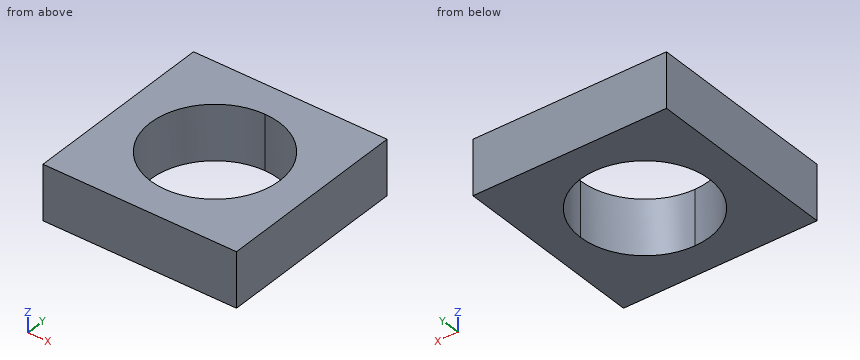
```python
from build123d import *

# Parameters (mm, degrees)
F1_DEPTH = 2.159


with BuildPart() as f1:
    # F0 (on Top) → F1 (new body)
    with BuildSketch(Plane.XY):
        with BuildLine():
            Line((-3.81, 0), (0, 0))
            Line((0, 0), (0, 1.27))
            ThreePointArc((0, 1.27), (-2.54, 3.81), (0, 6.35))
            Line((0, 6.35), (0, 7.62))
            Line((0, 7.62), (-3.81, 7.62))
            Line((-3.81, 7.62), (-3.81, 0))
        make_face()
        with BuildLine():
            Line((0, 1.27), (0, 0))
            Line((0, 0), (3.81, 0))
            Line((3.81, 0), (3.81, 7.62))
            Line((3.81, 7.62), (0, 7.62))
            Line((0, 7.62), (0, 6.35))
            ThreePointArc((0, 6.35), (1.796051, 5.606051), (2.54, 3.81))
            ThreePointArc((2.54, 3.81), (1.796051, 2.013949), (0, 1.27))
        make_face()
    extrude(amount=F1_DEPTH)


solid = f1.part
```
Could you check a few things on this model? Use its own coordinates, in mm. Round coordinates to 2 decimals unless told otherwise and drop trailing zeros. Loops run counter-clockwise (first coordinate to the right, second up) from the corner with the lowest first, then second, coordinate; pieces in that order, holes last.
Q1. I want a section at C-C (z = 1.5). Write out the boundary of the cut face in (x, y), and give its area (3 significant figures).
Q2. I want a section at B-B (x = 1). Write out the boundary of the cut face in (y, z).
Q3. Please list where these lines run through material, in increasing order: L1, parallel to Y at x = 0.5, z = 0.1; L2, parallel to X at y = 4.75, z = 0.55; L3, parallel to X at y = 3.75, z = 0.4.
Q4. I want a section at A-A (y = 3.5). Write out the boundary of the cut face in (x, z), and give its area (3 significant figures).
Answer below:
1. outline: (-3.81, 0) - (3.81, 0) - (3.81, 7.62) - (-3.81, 7.62) - close; hole (0, 6.35) arc R2.54 ccw (long way) to (2.54, 3.81) arc R2.54 ccw to start
1. area: 37.8 mm2
2. outline: (0, 0) - (1.48, 0) - (1.48, 2.16) - (0, 2.16) - close; (6.14, 0) - (7.62, 0) - (7.62, 2.16) - (6.14, 2.16) - close
3. L1: y = 0 to 1.32, 6.3 to 7.62
3. L2: x = -3.81 to -2.36, 2.36 to 3.81
3. L3: x = -3.81 to -2.54, 2.54 to 3.81
4. outline: (-3.81, 0) - (-2.52, 0) - (-2.52, 2.16) - (-3.81, 2.16) - close; (2.52, 0) - (3.81, 0) - (3.81, 2.16) - (2.52, 2.16) - close
4. area: 5.57 mm2
